The model under review builds one solid part; all positions refer to its coordinate system, in mm. A direction names the side the tool comes from. Coordinates: 2 decimals unless noted, no trailing zeros. Order: outer loops, then holes, each group sorted by start corner. A loop starts at its lowest first (then second) coordinate and runs counter-clockwise, first axis right, second up. Notation, with made-up numbers: M 76.25,49 L 125.25,49 A29 ccw 125.25,74 Z; hole C 46.25,-4 d11. An arc over 180 degrees is marked long. One line per item, written item: value.
```python
from build123d import *

# Parameters (mm, degrees)
SKETCH1_W           = 150
SKETCH1_H           = 380
SKETCH1_W_2         = 30
SKETCH1_H_2         = 8
SKETCH1_W_3         = 20
BOSS_EXTRUDE1_DEPTH = 8
SKETCH2_W           = 7.9
SKETCH2_H           = 30
BOSS_EXTRUDE2_DEPTH = 8
CUT_EXTRUDE2_DEPTH  = 9


with BuildPart() as part:
    # Sketch1 → Boss-Extrude1 (new body)
    with BuildSketch(Plane.XY):
        with Locations((75, 190)):
            Rectangle(SKETCH1_W, SKETCH1_H)
        with Locations((40, 154.566938385)):
            Rectangle(SKETCH1_W_2, SKETCH1_H_2, mode=Mode.SUBTRACT)
        with Locations((110, 154.566938385)):
            Rectangle(SKETCH1_W_2, SKETCH1_H_2, mode=Mode.SUBTRACT)
        with Locations((40, 26.566938385)):
            Rectangle(SKETCH1_W_2, SKETCH1_H_2, mode=Mode.SUBTRACT)
        with Locations((110, 26.566938385)):
            Rectangle(SKETCH1_W_2, SKETCH1_H_2, mode=Mode.SUBTRACT)
        with Locations((75, 9.5)):
            Rectangle(SKETCH1_W_3, SKETCH1_H_2, mode=Mode.SUBTRACT)
    extrude(amount=BOSS_EXTRUDE1_DEPTH)

    # Sketch2 → Boss-Extrude2 (add)
    with BuildSketch(Plane.XY.offset(8)):
        with Locations((153.95, 335)):
            Rectangle(SKETCH2_W, SKETCH2_H)
        with Locations((-3.95, 335)):
            Rectangle(SKETCH2_W, SKETCH2_H)
        with Locations((153.95, 275)):
            Rectangle(SKETCH2_W, SKETCH2_H)
        with Locations((-3.95, 275)):
            Rectangle(SKETCH2_W, SKETCH2_H)
        with Locations((153.95, 215)):
            Rectangle(SKETCH2_W, SKETCH2_H)
        with Locations((-3.95, 215)):
            Rectangle(SKETCH2_W, SKETCH2_H)
        with Locations((153.95, 155)):
            Rectangle(SKETCH2_W, SKETCH2_H)
        with Locations((-3.95, 155)):
            Rectangle(SKETCH2_W, SKETCH2_H)
        with Locations((153.95, 95)):
            Rectangle(SKETCH2_W, SKETCH2_H)
        with Locations((-3.95, 95)):
            Rectangle(SKETCH2_W, SKETCH2_H)
        with Locations((153.95, 35)):
            Rectangle(SKETCH2_W, SKETCH2_H)
        with Locations((-3.95, 35)):
            Rectangle(SKETCH2_W, SKETCH2_H)
    extrude(amount=-BOSS_EXTRUDE2_DEPTH)

    # Sketch3 → Cut-Extrude2 (cut, through all)
    with BuildSketch(Plane(origin=(0, 0, 0), x_dir=(-1, 0, 0), z_dir=(0, 0, -1))):
        with BuildLine():
            Line((-67.5, 25), (-82.5, 25))
            ThreePointArc((-82.5, 25), (-87.5, 30), (-82.5, 35))
            Line((-82.5, 35), (-67.5, 35))
            ThreePointArc((-67.5, 35), (-62.5, 30), (-67.5, 25))
        make_face()
        Polygon((7.9, 336.65), (4.3, 336.65), (4.3, 338.5), (2.1, 338.5), (2.1, 336.65), (0.1, 336.65), (0.1, 333.35), (2.1, 333.35), (2.1, 331.5), (4.3, 331.5), (4.3, 333.35), (7.9, 333.35), align=None)
        Polygon((-157.9, 213.35), (-154.3, 213.35), (-154.3, 211.5), (-152.1, 211.5), (-152.1, 213.35), (-150.1, 213.35), (-150.1, 216.65), (-152.1, 216.65), (-152.1, 218.5), (-154.3, 218.5), (-154.3, 216.65), (-157.9, 216.65), align=None)
        Polygon((-157.9, 273.35), (-154.3, 273.35), (-154.3, 271.5), (-152.1, 271.5), (-152.1, 273.35), (-150.1, 273.35), (-150.1, 276.65), (-152.1, 276.65), (-152.1, 278.5), (-154.3, 278.5), (-154.3, 276.65), (-157.9, 276.65), align=None)
        Polygon((7.9, 276.65), (4.3, 276.65), (4.3, 278.5), (2.1, 278.5), (2.1, 276.65), (0.1, 276.65), (0.1, 273.35), (2.1, 273.35), (2.1, 271.5), (4.3, 271.5), (4.3, 273.35), (7.9, 273.35), align=None)
        Polygon((7.9, 216.65), (4.3, 216.65), (4.3, 218.5), (2.1, 218.5), (2.1, 216.65), (0.1, 216.65), (0.1, 213.35), (2.1, 213.35), (2.1, 211.5), (4.3, 211.5), (4.3, 213.35), (7.9, 213.35), align=None)
        Polygon((-157.9, 333.35), (-154.3, 333.35), (-154.3, 331.5), (-152.1, 331.5), (-152.1, 333.35), (-150.1, 333.35), (-150.1, 336.65), (-152.1, 336.65), (-152.1, 338.5), (-154.3, 338.5), (-154.3, 336.65), (-157.9, 336.65), align=None)
        Polygon((0, 123.35), (0, 126.65), (-4, 126.65), (-4, 128.5), (-6.2, 128.5), (-6.2, 126.65), (-8.2, 126.65), (-8.2, 123.35), (-6.2, 123.35), (-6.2, 121.5), (-4, 121.5), (-4, 123.35), align=None)
        Polygon((0, 63.35), (0, 66.65), (-4, 66.65), (-4, 68.5), (-6.2, 68.5), (-6.2, 66.65), (-8.2, 66.65), (-8.2, 63.35), (-6.2, 63.35), (-6.2, 61.5), (-4, 61.5), (-4, 63.35), align=None)
        Polygon((-150, 63.35), (-146, 63.35), (-146, 61.5), (-143.8, 61.5), (-143.8, 63.35), (-141.8, 63.35), (-141.8, 66.65), (-143.8, 66.65), (-143.8, 68.5), (-146, 68.5), (-146, 66.65), (-150, 66.65), align=None)
        Polygon((-150, 123.35), (-146, 123.35), (-146, 121.5), (-143.8, 121.5), (-143.8, 123.35), (-141.8, 123.35), (-141.8, 126.65), (-143.8, 126.65), (-143.8, 128.5), (-146, 128.5), (-146, 126.65), (-150, 126.65), align=None)
    extrude(amount=-CUT_EXTRUDE2_DEPTH, mode=Mode.SUBTRACT)


solid = part.part
```
(1) We need section B-B, the plane z = 1.75. Count the separate pieces of the cut face and the enclosed holes in it, plus the area to 3 significant figures.
Geometry results:
separate pieces: 1
enclosed holes: 6
area: 58,200 mm2
(2) We need section A-A, the plane x = 50. State the section outline as (y, z) points.
Geometry results:
outline: M 0,0 L 22.57,0 L 22.57,8 L 0,8 Z; M 30.57,0 L 150.57,0 L 150.57,8 L 30.57,8 Z; M 158.57,0 L 380,0 L 380,8 L 158.57,8 Z
(3) Tool access review of faces 1 (the flat face through (-4, 290, 4)), 2 (the flat face through (154, 170, 4)), 3 (the flat face through (110, 30.567, 4)): name each direction out of +Z, -Z, +X, -X, +Y, -Y from which nothing blocks a thin tool from reaching the whole face with its end or side.
Geometry results:
face 1: +Z, -Z, -X
face 2: +Z, -Z, +X
face 3: +Z, -Z
(4) For L1, parallel to Y at x = 51, z = 6; L2, parallel to X at y = 273, z = 7.5; L3, parallel to Y at x = 8, z = 6, list the stretches that pass through material, from the lowest coordinate up.
Geometry results:
L1: y = 0 to 22.57, 30.57 to 150.57, 158.57 to 380
L2: x = -7.9 to -4.3, -2.1 to 152.1, 154.3 to 157.9
L3: y = 0 to 63.35, 66.65 to 123.35, 126.65 to 380
(5) Insertion check: pin 1 Ø0.7 at (x, z) = (153.5, 2.5) entering from +Y; pin 2 Ø1.5 at (y, z) = (122.5, 2.5) entering from +X; pin 3 Ø4 at (x, z) = (-5.5, 4) entering from -Y. Each pin has a flat end and moves straight along its axis. Give the tip position at first contact, or say it passes through.
Geometry results:
pin 1: stops at y = 350
pin 2: stops at x = 150
pin 3: stops at y = 20
(6) Mouldability with a two-part tool opening along Y and no side actions: class faces 4 (the flat face through (154, 350, 4)), 5 (the flat face through (154, 20, 4)), 6 (the flat face through (154, 50, 4)) as +Y half, -Y half, draft (parallel to the pull), parting line (faces both ways), or undercut.
Geometry results:
face 4: +Y half
face 5: -Y half
face 6: undercut
